Read the model definition and answer for the solid it produces. Units are mm, in the model's axes. A direction names the side the tool comes from. Coordinates: 2 decimals unless noted, no trailing zeros. Loops run counter-clockwise (first coordinate to the right, second up) from the corner with the lowest first, then second, coordinate; pieces in that order, holes last. Notation, with made-up numbers: (89, 49) -> (104, 49) arc R30 ccw to (104, 76) -> close; hole circle Ø2 at (-3, 28). An arc over 180 degrees is marked (long way). Answer as a JSON object with one key per item and string values. Group by question number.
1) Flat-ended cylindrical pins translate along their axes: P1, Ø1.5, axis at x = -8.5, z = 5.5, coming from the +Y side; P2, Ø1.5, axis at y = -30.5, z = 4, coming from the -X side. Find the tip coordinate at first contact, or state that the pin passes through.
2) Which of the six approach directions +Z, -Z, +X, -X, +Y, -Y give full straight-line access (tool end or side, diameter ignored) to faces 1 (the face through (2.956, 17.141, 3.451)), 2 (the face through (8, -8, 7))?
3) Section D-D, the plane x = -31 is taken. Give the vertices of the cut face in (y, z).
4) Section C-C, the plane y = 1.5 is taken. Give the vertices of the cut face in (x, z).
5) Section A-A, the plane x = 0 is taken. Give the vertices of the cut face in (y, z).
6) Consider probe 1 along Y at (x, z) = (0, 3.25); probe 2 along Y at (x, z) = (14.5, 6.5); probe 3 along X at (y, z) = (15, 1). Determine where each line is inside the solid, lowest interval first. Write a range as [from, to].
7) Section B-B, the plane z = 4 is taken. Count the separate pieces of the cut face and the enclosed holes in it, plus the area to 3 significant figures.
from build123d import *

# Parameters (mm, degrees)
F0_R     = 40
F0_R_2   = 35
F0_R_3   = 30
F0_R_4   = 11.15
F1_DEPTH = 7
F2_R     = 2


with BuildPart() as f1:
    # F0 (on Top) → F1 (new body)
    with BuildSketch(Plane.XY):
        Circle(F0_R)
        Circle(F0_R_2, mode=Mode.SUBTRACT)
        Circle(F0_R_2)
        Circle(F0_R_3, mode=Mode.SUBTRACT)
        Circle(F0_R_3)
        with BuildLine():
            ThreePointArc((0.1811274542, 24.9993438483), (14.6946313073, 20.2254248594), (23.7198174085, 7.8974845429))
            Line((23.7198174085, 7.8974845429), (24.2635492258, 7.883705044))
            Line((24.2635492258, 7.883705044), (23.8317603315, 7.5529596518))
            ThreePointArc((23.8317603315, 7.5529596518), (24.7062138772, 3.8213866405), (25, 0))
            ThreePointArc((25, 0), (22.3161322869, -11.2689946204), (14.8407808196, -20.1184299752))
            Line((14.8407808196, -20.1184299752), (14.9956981092, -20.6398077624))
            Line((14.9956981092, -20.6398077624), (14.5477104425, -20.3313580678))
            ThreePointArc((14.5477104425, -20.3313580678), (0, -25), (-14.5477104425, -20.3313580678))
            Line((-14.5477104425, -20.3313580678), (-14.9956981092, -20.6398077624))
            Line((-14.9956981092, -20.6398077624), (-14.8407808196, -20.1184299752))
            ThreePointArc((-14.8407808196, -20.1184299752), (-23.7764129074, -7.7254248594), (-23.8317603315, 7.5529596518))
            Line((-23.8317603315, 7.5529596518), (-24.2635492258, 7.883705044))
            Line((-24.2635492258, 7.883705044), (-23.7198174085, 7.8974845429))
            ThreePointArc((-23.7198174085, 7.8974845429), (-14.6946313073, 20.2254248594), (-0.1811274542, 24.9993438483))
            Line((-0.1811274542, 24.9993438483), (0, 25.5122054368))
            Line((0, 25.5122054368), (0.1811274542, 24.9993438483))
        make_face(mode=Mode.SUBTRACT)
        with BuildLine():
            Line((13.1343616929, -0.6411262894), (10.2490772421, 8.2388661651))
            ThreePointArc((10.2490772421, 8.2388661651), (7.7293760676, 10.638573476), (4.6684883087, 12.2934013565))
            Line((4.6684883087, 12.2934013565), (-4.6684883087, 12.2934013565))
            ThreePointArc((-4.6684883087, 12.2934013565), (-7.7293760676, 10.638573476), (-10.2490772421, 8.2388661651))
            Line((-10.2490772421, 8.2388661651), (-13.1343616929, -0.6411262894))
            ThreePointArc((-13.1343616929, -0.6411262894), (-12.5063931893, -4.063573476), (-11.0027663976, -7.2015020377))
            Line((-11.0027663976, -7.2015020377), (-3.4489936381, -12.6896391944))
            ThreePointArc((-3.4489936381, -12.6896391944), (0, -13.15), (3.4489936381, -12.6896391944))
            Line((3.4489936381, -12.6896391944), (11.0027663976, -7.2015020377))
            ThreePointArc((11.0027663976, -7.2015020377), (12.5063931893, -4.063573476), (13.1343616929, -0.6411262894))
        make_face()
        Circle(F0_R_4, mode=Mode.SUBTRACT)
        with BuildLine():
            ThreePointArc((-4.6684883087, 12.2934013565), (0, 13.15), (4.6684883087, 12.2934013565))
            Line((4.6684883087, 12.2934013565), (0.1811274542, 24.9993438483))
            ThreePointArc((0.1811274542, 24.9993438483), (0, 25), (-0.1811274542, 24.9993438483))
            Line((-0.1811274542, 24.9993438483), (-4.6684883087, 12.2934013565))
        make_face()
        with BuildLine():
            ThreePointArc((-13.1343616929, -0.6411262894), (-12.5063931893, 4.063573476), (-10.2490772421, 8.2388661651))
            Line((-10.2490772421, 8.2388661651), (-23.7198174085, 7.8974845429))
            ThreePointArc((-23.7198174085, 7.8974845429), (-23.7764129074, 7.7254248594), (-23.8317603315, 7.5529596518))
            Line((-23.8317603315, 7.5529596518), (-13.1343616929, -0.6411262894))
        make_face()
        with BuildLine():
            Line((-14.5477104425, -20.3313580678), (-3.4489936381, -12.6896391944))
            ThreePointArc((-3.4489936381, -12.6896391944), (-7.7293760676, -10.638573476), (-11.0027663976, -7.2015020377))
            Line((-11.0027663976, -7.2015020377), (-14.8407808196, -20.1184299752))
            ThreePointArc((-14.8407808196, -20.1184299752), (-14.6946313073, -20.2254248594), (-14.5477104425, -20.3313580678))
        make_face()
        with BuildLine():
            Line((14.8407808196, -20.1184299752), (11.0027663976, -7.2015020377))
            ThreePointArc((11.0027663976, -7.2015020377), (7.7293760676, -10.638573476), (3.4489936381, -12.6896391944))
            Line((3.4489936381, -12.6896391944), (14.5477104425, -20.3313580678))
            ThreePointArc((14.5477104425, -20.3313580678), (14.6946313073, -20.2254248594), (14.8407808196, -20.1184299752))
        make_face()
        with BuildLine():
            ThreePointArc((10.2490772421, 8.2388661651), (12.4035854843, 4.3673295197), (13.15, 0))
            ThreePointArc((13.15, 0), (13.1460898419, -0.3206584927), (13.1343616929, -0.6411262894))
            Line((13.1343616929, -0.6411262894), (23.8317603315, 7.5529596518))
            ThreePointArc((23.8317603315, 7.5529596518), (23.7764129074, 7.7254248594), (23.7198174085, 7.8974845429))
            Line((23.7198174085, 7.8974845429), (10.2490772421, 8.2388661651))
        make_face()
        with BuildLine():
            Line((-4.6684883087, 12.2934013565), (4.6684883087, 12.2934013565))
            ThreePointArc((4.6684883087, 12.2934013565), (0, 13.15), (-4.6684883087, 12.2934013565))
        make_face()
        with BuildLine():
            ThreePointArc((13.1343616929, -0.6411262894), (13.1460898419, -0.3206584927), (13.15, 0))
            ThreePointArc((13.15, 0), (12.4035854843, 4.3673295197), (10.2490772421, 8.2388661651))
            Line((10.2490772421, 8.2388661651), (13.1343616929, -0.6411262894))
        make_face()
        with BuildLine():
            ThreePointArc((3.4489936381, -12.6896391944), (7.7293760676, -10.638573476), (11.0027663976, -7.2015020377))
            Line((11.0027663976, -7.2015020377), (3.4489936381, -12.6896391944))
        make_face()
        with BuildLine():
            ThreePointArc((-11.0027663976, -7.2015020377), (-7.7293760676, -10.638573476), (-3.4489936381, -12.6896391944))
            Line((-3.4489936381, -12.6896391944), (-11.0027663976, -7.2015020377))
        make_face()
        with BuildLine():
            Line((-13.1343616929, -0.6411262894), (-10.2490772421, 8.2388661651))
            ThreePointArc((-10.2490772421, 8.2388661651), (-12.5063931893, 4.063573476), (-13.1343616929, -0.6411262894))
        make_face()
        with BuildLine():
            ThreePointArc((-23.8317603315, 7.5529596518), (-23.7764129074, 7.7254248594), (-23.7198174085, 7.8974845429))
            Line((-23.7198174085, 7.8974845429), (-24.2635492258, 7.883705044))
            Line((-24.2635492258, 7.883705044), (-23.8317603315, 7.5529596518))
        make_face()
        with BuildLine():
            Line((-14.9956981092, -20.6398077624), (-14.5477104425, -20.3313580678))
            ThreePointArc((-14.5477104425, -20.3313580678), (-14.6946313073, -20.2254248594), (-14.8407808196, -20.1184299752))
            Line((-14.8407808196, -20.1184299752), (-14.9956981092, -20.6398077624))
        make_face()
        with BuildLine():
            Line((14.9956981092, -20.6398077624), (14.8407808196, -20.1184299752))
            ThreePointArc((14.8407808196, -20.1184299752), (14.6946313073, -20.2254248594), (14.5477104425, -20.3313580678))
            Line((14.5477104425, -20.3313580678), (14.9956981092, -20.6398077624))
        make_face()
        with BuildLine():
            Line((24.2635492258, 7.883705044), (23.7198174085, 7.8974845429))
            ThreePointArc((23.7198174085, 7.8974845429), (23.7764129074, 7.7254248594), (23.8317603315, 7.5529596518))
            Line((23.8317603315, 7.5529596518), (24.2635492258, 7.883705044))
        make_face()
        with BuildLine():
            ThreePointArc((-0.1811274542, 24.9993438483), (0, 25), (0.1811274542, 24.9993438483))
            Line((0.1811274542, 24.9993438483), (0, 25.5122054368))
            Line((0, 25.5122054368), (-0.1811274542, 24.9993438483))
        make_face()
    extrude(amount=F1_DEPTH)

    # F2
    f2_edges = [f1.edges().sort_by_distance(p)[0] for p in [
        (0.181127, 24.999344, 3.5),
        (-0.181127, 24.999344, 3.5),
        (23.719817, 7.897485, 3.5),
        (23.83176, 7.55296, 3.5),
        (14.840781, -20.11843, 3.5),
        (14.54771, -20.331358, 3.5),
        (-14.54771, -20.331358, 3.5),
        (-14.840781, -20.11843, 3.5),
        (-23.83176, 7.55296, 3.5),
        (-23.719817, 7.897485, 3.5),
    ]]
    fillet(f2_edges, radius=F2_R)


solid = f1.part
Determined:
{
 "1": {"P1": "y = 39.24", "P2": "x = -26.74"},
 "2": {"face 1": "+Z, -Z", "face 2": "+Z, +X, -X, +Y, -Y"},
 "3": {"outline": "(-25.28, 0) -> (25.28, 0) -> (25.28, 7) -> (-25.28, 7) -> close"},
 "4": {"outline": "(-39.97, 0) -> (-24.95, 0) -> (-24.95, 7) -> (-39.97, 7) -> close; (-15.93, 0) -> (-11.05, 0) -> (-11.05, 7) -> (-15.93, 7) -> close; (11.05, 0) -> (15.93, 0) -> (15.93, 7) -> (11.05, 7) -> close; (24.95, 0) -> (39.97, 0) -> (39.97, 7) -> (24.95, 7) -> close"},
 "5": {"outline": "(-40, 0) -> (-25, 0) -> (-25, 7) -> (-40, 7) -> close; (-13.15, 0) -> (-11.15, 0) -> (-11.15, 7) -> (-13.15, 7) -> close; (11.15, 0) -> (40, 0) -> (40, 7) -> (11.15, 7) -> close"},
 "6": {"probe 1": "[-40, -25], [-13.15, -11.15], [11.15, 40]", "probe 2": "[-37.28, -18.07], [0.4, 8.13], [20.37, 37.28]", "probe 3": "[-37.08, -20], [-3.71, 3.71], [20, 37.08]"},
 "7": {"separate pieces": "1", "enclosed holes": "6", "area": "3,520 mm²"}
}
